Part model, mm, in its own coordinate system. Face numbers are marked on the shaded views. A direction names the side the tool comes from. Give positions to 0.01 mm unless a question says otherwise; leave off trailing zeros. Write each loop counter-clockwise with the first axis right and the second up, starting at its lowest first coordinate (ties: lowest second). Pieces come first, ordered by that corner, then holes. Notation, with made-up numbers: M -26,-8 L 27,-8 A17 ccw 27,7 Z; hole C 43,63 d10. An arc over 180 degrees is marked long. Use a Markdown table: item, result.
```python
from build123d import *

# Parameters (mm, degrees)
F2_SIZE = 2.54
F3_R    = 1.5875


with BuildPart() as f1:
    # F0 (on Front) → F1 (revolve)
    with BuildSketch(Plane.XZ):
        Polygon((8.6614, 14.962643), (0, 14.962643), (0, -10.437357), (19.05, -10.437357), (19.05, 0.990691), (15.875, 0.990691), (8.6614, 2.262643), align=None)
    revolve(axis=Axis((0, 0, 1.824711), (0, 0, -1)))

    # F2
    f2_edges = [f1.edges().sort_by_distance(p)[0] for p in [
        (-8.6614, 0, 14.962643),
    ]]
    chamfer(f2_edges, length=F2_SIZE)

    # F3
    f3_edges = [f1.edges().sort_by_distance(p)[0] for p in [
        (-19.05, 0, -10.437357),
    ]]
    fillet(f3_edges, radius=F3_R)


solid = f1.part
```
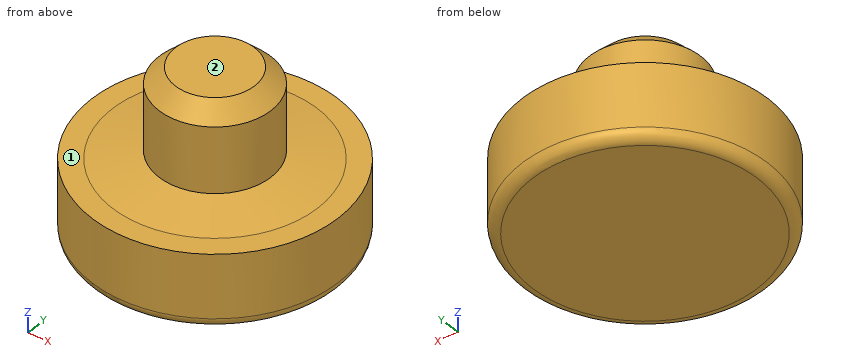
1. Drill centre lines: L1, parallel to Z at x = 12, y = 11; L2, parallel to Y at x = 5, z = -7.75; L3, parallel to X at y = 0, z = -9. Where is each one in solid material? Low to high.
Findings below:
| item | result |
|---|---|
| L1 | -10.44 to 0.99 |
| L2 | -18.38 to 18.38 |
| L3 | -19.04 to 19.04 |
2. Cut at D-D, the plane z = 7. Give the cut face in (x, y), then the cut area to 3 significant figures.
Findings below:
| item | result |
|---|---|
| outline | C 0,0 d17.32 |
| area | 236 mm2 |
3. Drop flat-ended pins along their axis: P1, Ø4, axis at x = 12.5, z = 0.5, coming from the +Y side; P2, Ø5, axis at x = 6, y = 12.5, coming from the +Z side; P3, Ø12, axis at x = 12.5, z = -0.5, coming from the -Y side. Give the stop position or say it passes through.
Findings below:
| item | result |
|---|---|
| P1 | y = 15.9 |
| P2 | z = 1.79 |
| P3 | y = -17.91 |
4. Tool access for the marked faces 1 and 2: list every direction of +Z, -Z, +X, -X, +Y, -Y with a clear straight run to the whole face (end or side of a thin tool).
Findings below:
| item | result |
|---|---|
| face 1 | +Z |
| face 2 | +Z, +X, -X, +Y, -Y |
5. Cut at C-C, the plane z = -5. Give the cut face in (x, y).
Findings below:
| item | result |
|---|---|
| outline | C 0,0 d38.1 |
